Build history of the part. All positions in model axes, mm. A direction names the side the tool comes from. Coordinates: 2 decimals unless noted, no trailing zeros.
Item 1: Mould opens along Z. For faces 1 (the face through (103, 37, -466)), 2 (the face through (100, 21, -920)), 3 (the face through (15.249, 31.577, -50.214)) say: released by +Z, released by -Z, zero draft, split by the parting line, or undercut.
Item 2: 3-axis set-ups, long thin cutter, end or side, ignore diameter. For faces 4 (the face through (15.249, 31.577, -790.214)), 5 (the face through (0, 21, -454)): which of +Z, -Z, +X, -X, +Y, -Y reach the whole face in a straight line?
Item 3: Cut at A-A (y = 32). Count the separate pieces of the cut face and the enclosed holes in it, and give its area (3 significant figures).
Item 4: Flat gauge pins, fed straight in: pin 1 (16 mm diameter, centred on x = 99.2, z = -59, fed in from +Y); pin 2 (3 mm diameter, centred on x = 10.2, z = -225, fed in from +Y); pin 3 (11 mm diameter, centred on x = 10.2, z = -225, fed in from +Y). Where does each tip first touch, or does it go through?
Item 5: Drill centre lines: line 1 along Z through (x, y) = (10.2, 11.25); line 2 along X through (y, z) = (25, -602); line 3 along Z through (x, y) = (141.2, 31.5). Where is each one in solid material? Low to high.
from build123d import *

# Parameters (mm, degrees)
SKETCH1_W                                            = 203.2
SKETCH1_H                                            = 920
BOSS_EXTRUDE1_DEPTH                                  = 50.8
SKETCH2_W                                            = 203.2
SKETCH2_H                                            = 5
CUT_EXTRUDE1_DEPTH                                   = 944.541668396
SKETCH6_W                                            = 256
SKETCH6_H                                            = 13.8
CUT_EXTRUDE3_DEPTH                                   = 944.541668396
M12_CLEARANCE_HOLE1_D                                = 13.5
CBORE_FOR_M10_HEX_SOCKET_HEAD_CAP_SCREW1_D           = 11
CBORE_FOR_M10_HEX_SOCKET_HEAD_CAP_SCREW1_CBORE_D     = 18
CBORE_FOR_M10_HEX_SOCKET_HEAD_CAP_SCREW1_CBORE_DEPTH = 11
M6_TAPPED_HOLE1_D                                    = 5
M6_TAPPED_HOLE1_DEPTH                                = 27.99
M6_TAPPED_HOLE1_TIP                                  = 1.502151548
M6_TAPPED_HOLE2_D                                    = 5
M6_TAPPED_HOLE2_DEPTH                                = 27.99
M6_TAPPED_HOLE2_TIP                                  = 1.502151548
F_13_5_13_5_DIAMETER_HOLE1_D                         = 13.5
F_13_5_13_5_DIAMETER_HOLE1_DEPTH                     = 20
F_13_5_13_5_DIAMETER_HOLE1_TIP                       = 4.055809178
M10_TAPPED_HOLE1_D                                   = 8.5
M10_TAPPED_HOLE1_DEPTH                               = 38
M10_TAPPED_HOLE1_TIP                                 = 2.553657631


with BuildPart() as part:
    # Sketch1 → Boss-Extrude1 (new body)
    with BuildSketch(Plane(origin=(0, 0, 0), x_dir=(1, 0, 0), z_dir=(0, 1, 0))):
        with Locations((101.6, 460)):
            Rectangle(SKETCH1_W, SKETCH1_H)
    extrude(amount=BOSS_EXTRUDE1_DEPTH)

    # Sketch2 → Cut-Extrude1 (cut, through all)
    with BuildSketch(Plane(origin=(0, 0, -920), x_dir=(-1, 0, 0), z_dir=(0, 0, -1))):
        with Locations((-101.6, 2.5)):
            Rectangle(SKETCH2_W, SKETCH2_H)
    extrude(amount=-CUT_EXTRUDE1_DEPTH, mode=Mode.SUBTRACT)

    # Sketch6 → Cut-Extrude3 (cut, through all)
    with BuildSketch(Plane(origin=(0, 0, -920), x_dir=(-1, 0, 0), z_dir=(0, 0, -1))):
        with Locations((-75.2, 43.9)):
            Rectangle(SKETCH6_W, SKETCH6_H)
    extrude(amount=-CUT_EXTRUDE3_DEPTH, mode=Mode.SUBTRACT)

    # M12 Clearance Hole1 (through all)
    with Locations(Plane(origin=(7.928034887, 37, -192.870856327), x_dir=(-1, 0, 0), z_dir=(0, 1, 0))):
        with Locations((-170.271965113, 162.870856327), (-170.271965113, -697.129143673), (-170.271965113, -637.129143673), (-170.271965113, -547.129143673), (-170.271965113, -467.129143673), (-170.271965113, -307.129143673), (-170.271965113, -147.129143673), (-170.271965113, -67.129143673), (-170.271965113, 102.870856327), (-170.271965113, -387.129143673), (-170.271965113, -227.129143673), (-170.271965113, 12.870856327)):
            Hole(M12_CLEARANCE_HOLE1_D / 2)

    # CBORE for M10 Hex Socket Head Cap Screw1 (through all)
    with Locations(Plane(origin=(-145.411860995, 37, -401.636592577), x_dir=(1, 0, 0), z_dir=(0, 1, 0))):
        with Locations((162.611860995, -280.636592577), (244.611860995, -342.636592577), (162.611860995, -342.636592577), (244.611860995, -280.636592577), (162.611860995, 459.363407423), (244.611860995, 397.363407423), (162.611860995, 397.363407423), (244.611860995, 459.363407423)):
            CounterBoreHole(CBORE_FOR_M10_HEX_SOCKET_HEAD_CAP_SCREW1_D / 2, CBORE_FOR_M10_HEX_SOCKET_HEAD_CAP_SCREW1_CBORE_D / 2, CBORE_FOR_M10_HEX_SOCKET_HEAD_CAP_SCREW1_CBORE_DEPTH)

    # M6 Tapped Hole1
    with Locations(Plane.XZ.offset(-5)):
        with Locations((10.2, -720), (10.2, -695), (10.2, -200), (10.2, -225)):
            Hole(M6_TAPPED_HOLE1_D / 2, depth=M6_TAPPED_HOLE1_DEPTH)
            with Locations((0, 0, -(M6_TAPPED_HOLE1_DEPTH + M6_TAPPED_HOLE1_TIP / 2))):  # 118° drill point
                Cone(0, M6_TAPPED_HOLE1_D / 2, M6_TAPPED_HOLE1_TIP, mode=Mode.SUBTRACT)

    # M6 Tapped Hole2
    with Locations(Plane(origin=(0, 37, 0), x_dir=(1, 0, 0), z_dir=(0, 1, 0))):
        with Locations((141.2, 560), (183.2, 602), (141.2, 602), (183.2, 560)):
            Hole(M6_TAPPED_HOLE2_D / 2, depth=M6_TAPPED_HOLE2_DEPTH)
            with Locations((0, 0, -(M6_TAPPED_HOLE2_DEPTH + M6_TAPPED_HOLE2_TIP / 2))):  # 118° drill point
                Cone(0, M6_TAPPED_HOLE2_D / 2, M6_TAPPED_HOLE2_TIP, mode=Mode.SUBTRACT)

    # Ø13.5 (13.5) Diameter Hole1
    with Locations(Plane(origin=(0, 37, 0), x_dir=(1, 0, 0), z_dir=(0, 1, 0))):
        with Locations((10.2, 720), (10.2, 695), (10.2, 225), (10.2, 200)):
            Hole(F_13_5_13_5_DIAMETER_HOLE1_D / 2, depth=F_13_5_13_5_DIAMETER_HOLE1_DEPTH)
            with Locations((0, 0, -(F_13_5_13_5_DIAMETER_HOLE1_DEPTH + F_13_5_13_5_DIAMETER_HOLE1_TIP / 2))):  # 118° drill point
                Cone(0, F_13_5_13_5_DIAMETER_HOLE1_D / 2, F_13_5_13_5_DIAMETER_HOLE1_TIP, mode=Mode.SUBTRACT)

    # M10 Tapped Hole1
    with Locations(Plane(origin=(0, 37, 0), x_dir=(1, 0, 0), z_dir=(0, 1, 0))):
        with Locations((23, 164.5), (23, 260.5), (23, 508), (23, 412)):
            Hole(M10_TAPPED_HOLE1_D / 2, depth=M10_TAPPED_HOLE1_DEPTH)
            with Locations((0, 0, -(M10_TAPPED_HOLE1_DEPTH + M10_TAPPED_HOLE1_TIP / 2))):  # 118° drill point
                Cone(0, M10_TAPPED_HOLE1_D / 2, M10_TAPPED_HOLE1_TIP, mode=Mode.SUBTRACT)


solid = part.part
Filled sheet:
1. face 1: zero draft
1. face 2: released by -Z
1. face 3: undercut
2. face 4: +Y
2. face 5: +Z, -Z, -X, +Y, -Y
3. separate pieces: 1
3. enclosed holes: 32
3. area: 182,000 mm2
4. pin 1: stops at y = 26
4. pin 2: passes through
4. pin 3: stops at y = 16.25
5. line 1: z = -920 to -722.5, -717.5 to -697.5, -692.5 to -227.5, -222.5 to -202.5, -197.5 to 0
5. line 2: x = 0 to 138.7, 143.7 to 180.7, 185.7 to 203.2
5. line 3: z = -920 to -604.5, -599.5 to -562.5, -557.5 to 0
